Geometry check sheet. Reference: the model listing, model coordinates, mm. Coordinates: 2 decimals unless noted, no trailing zeros. Write each loop counter-clockwise with the first axis right and the second up, starting at its lowest first coordinate (ties: lowest second). Pieces come first, ordered by that corner, then holes. Notation, with made-up numbers: (-34.75, 39) -> (-30.75, 39) arc R25 cw to (-30.75, 78) -> close; hole circle Ø2 at (79, 56). An arc over 180 degrees is marked (long way). Answer in a Markdown table with one row per item. Add a question column.
1. Scan lines: L1, parallel to Y at x = 27.5, z = 0.7; L2, parallel to X at y = -1.5, z = 2.4; L3, parallel to X at y = -11.5, z = 0.65. Record each from-to range of solid material in increasing order. Write a range as from..to.
2. Cross-section at C-C on x = 27.5. Record the cut outline in (y, z), and give its area (3 significant figures).
3. Cross-section at D-D on x = -30. Record the cut outline in (y, z), and give its area (3 significant figures).
4. Cross-section at A-A on y = 0. Record the cut outline in (x, z), and give its area (3 significant figures).
5. Cross-section at B-B on z = 0.95. Record the cut outline in (x, y).
6. Mould release check, pull along Y, two halves, no side actions. Record for faces 1 (the cylindrical face through (-32.15, 11.99, 1.48)), 2 (the cylindrical face through (-29.25, 0.08, 1.52)), 3 (the flat face through (0, 0, 3)), 4 (the cylindrical face through (32.15, -11.99, 1.48)): pulls with the +Y half, pulls with the -Y half, needs draft (parallel to the pull), parting line crosses it, or undercut.
7. Depth check by flat-ended pin: P1, Ø4, axis at x = -21.5, y = -9, coming from the -Z side; P2, Ø2, axis at x = 27.5, y = 0, coming from the -Z side; P3, Ø1.5, axis at y = 6, z = 0.5, coming from the +X side. Enter the tip coordinate at first touch or a pass-through.
```python
from build123d import *

# Parameters (mm, degrees)
BOSS_EXTRUDE1_DEPTH = 3
SKETCH2_R           = 1.75
CUT_EXTRUDE1_DEPTH  = 3


with BuildPart() as part:
    # Sketch1 → Boss-Extrude1 (new body)
    with BuildSketch(Plane.XY):
        with BuildLine():
            Line((-25, 15), (25, 15))
            ThreePointArc((25, 15), (32.071067812, 12.071067812), (35, 5))
            Line((35, 5), (35, -5))
            ThreePointArc((35, -5), (32.071067812, -12.071067812), (25, -15))
            Line((25, -15), (-25, -15))
            ThreePointArc((-25, -15), (-32.071067812, -12.071067812), (-35, -5))
            Line((-35, -5), (-35, 5))
            ThreePointArc((-35, 5), (-32.071067812, 12.071067812), (-25, 15))
        make_face()
    extrude(amount=BOSS_EXTRUDE1_DEPTH)

    # Sketch2 → Cut-Extrude1 (cut)
    with BuildSketch(Plane.XY.offset(3)):
        with Locations((-27.5, 0)):
            Circle(SKETCH2_R)
        with Locations((27.5, 0)):
            Circle(SKETCH2_R)
    extrude(amount=-CUT_EXTRUDE1_DEPTH, mode=Mode.SUBTRACT)


solid = part.part
```
Results found:
| question | item | result |
|---|---|---|
| 1 | L1 | y = -14.68..-1.75, 1.75..14.68 |
| 1 | L2 | x = -35..-28.4, -26.6..26.6, 28.4..35 |
| 1 | L3 | x = -32.6..32.6 |
| 2 | outline | (-14.68, 0) -> (-1.75, 0) -> (-1.75, 3) -> (-14.68, 3) -> close; (1.75, 0) -> (14.68, 0) -> (14.68, 3) -> (1.75, 3) -> close |
| 2 | area | 77.6 mm^2 |
| 3 | outline | (-13.66, 0) -> (13.66, 0) -> (13.66, 3) -> (-13.66, 3) -> close |
| 3 | area | 82.0 mm^2 |
| 4 | outline | (-35, 0) -> (-29.25, 0) -> (-29.25, 3) -> (-35, 3) -> close; (-25.75, 0) -> (25.75, 0) -> (25.75, 3) -> (-25.75, 3) -> close; (29.25, 0) -> (35, 0) -> (35, 3) -> (29.25, 3) -> close |
| 4 | area | 189 mm^2 |
| 5 | outline | (-35, -5) arc R10 ccw to (-25, -15) -> (25, -15) arc R10 ccw to (35, -5) -> (35, 5) arc R10 ccw to (25, 15) -> (-25, 15) arc R10 ccw to (-35, 5) -> close; hole circle Ø3.5 at (-27.5, 0); hole circle Ø3.5 at (27.5, 0) |
| 6 | face 1 | pulls with the +Y half |
| 6 | face 2 | undercut |
| 6 | face 3 | needs draft |
| 6 | face 4 | pulls with the -Y half |
| 7 | P1 | stops at z = 0 |
| 7 | P2 | passes through |
| 7 | P3 | stops at x = 35 |
